Check sheet for the modelled part. Datum: model origin and axes. Units: mm. Face numbers are marked on the shaded views. A direction names the side the tool comes from. Round coordinates to 2 decimals unless told otherwise and drop trailing zeros. Write each loop counter-clockwise with the first axis right and the second up, starting at its lowest first coordinate (ties: lowest second). Pieces come first, ordered by that corner, then holes.
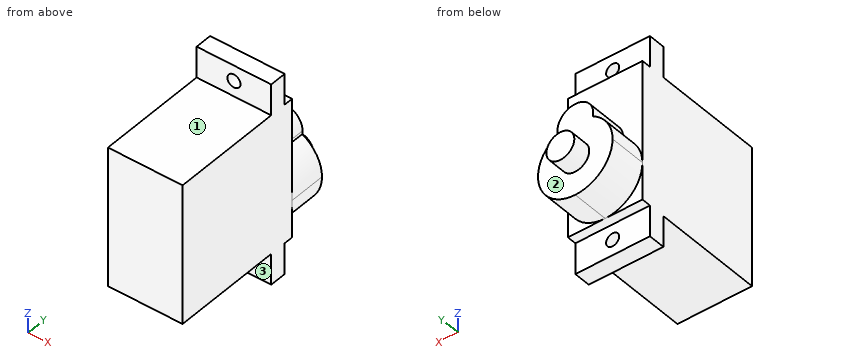
from build123d import *

# Parameters (mm, degrees)
SKETCH1_W           = 5
SKETCH1_H           = 2.7
SKETCH1_W_2         = 14.75
SKETCH1_H_2         = 6
BOSS_EXTRUDE1_DEPTH = 12
CUT_EXTRUDE1_DEPTH  = 6
SKETCH3_R           = 1.05
CUT_EXTRUDE2_DEPTH  = 2.7
SKETCH4_R           = 2.25
BOSS_EXTRUDE3_DEPTH = 3


with BuildPart() as part:
    # Sketch1 → Boss-Extrude1 (new body)
    with BuildSketch(Plane(origin=(0, 0, 0), x_dir=(0, 0, -1), z_dir=(1, 0, 0))):
        Polygon((-11.25, 6.8), (-11.25, -11), (11.25, -11), (11.25, 6.8), (11.25, 9.5), (11.25, 11), (-3.5, 11), (-11.25, 11), (-11.25, 9.5), align=None)
        with Locations((-13.75, 8.15)):
            Rectangle(SKETCH1_W, SKETCH1_H)
        with Locations((13.75, 8.15)):
            Rectangle(SKETCH1_W, SKETCH1_H)
        with Locations((3.875, 14)):
            Rectangle(SKETCH1_W_2, SKETCH1_H_2)
    extrude(amount=BOSS_EXTRUDE1_DEPTH)

    # Sketch2 → Cut-Extrude1 (cut)
    with BuildSketch(Plane(origin=(0, 17, 0), x_dir=(1, 0, 0), z_dir=(0, 1, 0))):
        with BuildLine():
            ThreePointArc((0, 5.25), (1.757359313, 9.492640687), (6, 11.25))
            Line((6, 11.25), (0, 11.25))
            Line((0, 11.25), (0, 5.25))
        make_face()
        with BuildLine():
            Line((12, 11.25), (6, 11.25))
            ThreePointArc((6, 11.25), (10.242640687, 9.492640687), (12, 5.25))
            Line((12, 5.25), (12, 11.25))
        make_face()
        with BuildLine():
            Line((12, -3.5), (12, 5.25))
            ThreePointArc((12, 5.25), (11.142901339, 2.159601026), (8.81647806, -0.04787234))
            ThreePointArc((8.81647806, -0.04787234), (8.860332098, -0.334956403), (8.875, -0.625))
            ThreePointArc((8.875, -0.625), (8.032931996, -2.657931996), (6, -3.5))
            Line((6, -3.5), (12, -3.5))
        make_face()
        with BuildLine():
            ThreePointArc((3.18352194, -0.04787234), (0.857098661, 2.159601026), (0, 5.25))
            Line((0, 5.25), (0, -3.5))
            Line((0, -3.5), (6, -3.5))
            ThreePointArc((6, -3.5), (3.772347983, -2.442468429), (3.18352194, -0.04787234))
        make_face()
    extrude(amount=-CUT_EXTRUDE1_DEPTH, mode=Mode.SUBTRACT)

    # Sketch3 → Cut-Extrude2 (cut)
    with BuildSketch(Plane(origin=(0, 9.5, 0), x_dir=(1, 0, 0), z_dir=(0, 1, 0))):
        with Locations(Location((6, -13.75, 0), (0, 0, 270))):
            Circle(SKETCH3_R)
        with Locations(Location((6, 13.75, 0), (0, 0, 270))):
            Circle(SKETCH3_R)
    extrude(amount=-CUT_EXTRUDE2_DEPTH, mode=Mode.SUBTRACT)

    # Sketch4 → Boss-Extrude3 (add)
    with BuildSketch(Plane(origin=(0, 17, 0), x_dir=(1, 0, 0), z_dir=(0, 1, 0))):
        with Locations(Location((6, 5.25, 0), (0, 0, 270))):
            Circle(SKETCH4_R)
    extrude(amount=BOSS_EXTRUDE3_DEPTH)


solid = part.part
1. Set-up check for the marked faces 1, 2 and 3: record each of +Z, -Z, +X, -X, +Y, -Y from which the full face is reachable in a straight line by a thin tool's end or side.
2. Sectioned sample at B-B, the plane y = 7.5. Enter the section's corners in (x, z), plus the area to 3 significant figures.
3. Sectioned sample at C-C, the plane y = 15. Enter the section's corners in (x, z) (3 decimals).
4. Scan lines: line 1 along X through (y, z) = (8.1, 13.75); line 2 along Y through (x, z) = (9.25, 3); line 3 along Y through (x, z) = (0.5, 13). Record each from-to range of solid material in increasing order.
5. Sectioned sample at D-D, the plane x = 10.5. Enter the section's corners in (y, z), plus the area to 3 significant figures.
6. Go/stop test with flat-tipped pins: pin 1 (1.9 mm diameter, centred on x = 6, z = 13.75, fed in from -Y); pin 2 (1 mm diameter, centred on x = 4, z = -11.5, fed in from -Y); pin 3 (4 mm diameter, centred on x = 9, z = 14.5, fed in from -Y); pin 4 (1.5 mm diameter, centred on x = 3.5, z = 13, fed in from +Y). Record where each tip stops, or that it passes through.
7. Sectioned sample at A-A, the plane z = -13.75. Enter the section's corners in (x, y).
Computed values:
1. face 1: +Z, +X, -X, -Y
1. face 2: +Y
1. face 3: -Z, +X, -X, -Y
2. outline: (0, -16.25) - (12, -16.25) - (12, 16.25) - (0, 16.25) - close; hole circle Ø2.1 at (6, -13.75); hole circle Ø2.1 at (6, 13.75)
2. area: 383 mm2
3. outline: (3.184, 0.048) arc R6 ccw (long way) to (8.816, 0.048) arc R2.875 ccw (long way) to start
4. line 1: x = 0 to 4.95, 7.05 to 12
4. line 2: y = -11 to 11
4. line 3: y = 6.8 to 9.5
5. outline: (-11, -11.25) - (6.8, -11.25) - (6.8, -16.25) - (9.5, -16.25) - (9.5, -11.25) - (11, -11.25) - (11, -9.22) - (17, -9.22) - (17, -1.28) - (11, -1.28) - (11, 11.25) - (9.5, 11.25) - (9.5, 16.25) - (6.8, 16.25) - (6.8, 11.25) - (-11, 11.25) - close
5. area: 570 mm2
6. pin 1: passes through
6. pin 2: stops at y = -11
6. pin 3: stops at y = 6.8
6. pin 4: stops at y = 9.5
7. outline: (0, 6.8) - (4.95, 6.8) - (4.95, 9.5) - (0, 9.5) - close; (7.05, 6.8) - (12, 6.8) - (12, 9.5) - (7.05, 9.5) - close
